Source: three-view drawing plus pictorial views. Frame: mm from the lowest corner of the part. Give positions to 0.01 mm unless a question says otherwise; leave off trailing zeros. Order: outer loops, then holes, each group sorted by start corner. A loop starts at its lowest first (then second) coordinate and runs counter-clockwise, first axis right, second up.
1) First-contact query: P1, Ø13, axis at x = 14.86, z = 35, coming from the +Y side; P2, Ø6, axis at y = 12.5, z = 46, coming from the -X side; P3, Ø10, axis at x = 17.5, y = 14.5, coming from the +Z side; P4, Ø1.5, axis at x = 50, z = 30, coming from the +Y side. Flat tips, straight axial feed; report the tip coordinate or a pass-through.
2) Section C-C, the plane x = 11.5. Return loops of the section in (y, z) (1 decimal).
3) Section B-B, the plane z = 58. Return loops of the section in (x, y) (1 decimal), plus the area to 3 significant figures.
4) Draft query along X for the marked faces 1, 2 and 3. Return one class per face: released by +X, released by -X, zero draft, split by the parting line, or undercut.
5) Section D-D, the plane y = 9.5. Return loops of the section in (x, z) (1 decimal).
6) Section A-A, the plane x = 33.5. Return loops of the section in (y, z) (1 decimal), plus the area to 3 significant figures.
7) Material intervals for line 1 (X direction, y = 11.25, z = 28) (1 decimal); line 2 (Y direction, x = 5, z = 45.5) (1 decimal); line 3 (X direction, y = 8.5, z = 47.5) (1 decimal), sorted ascending.
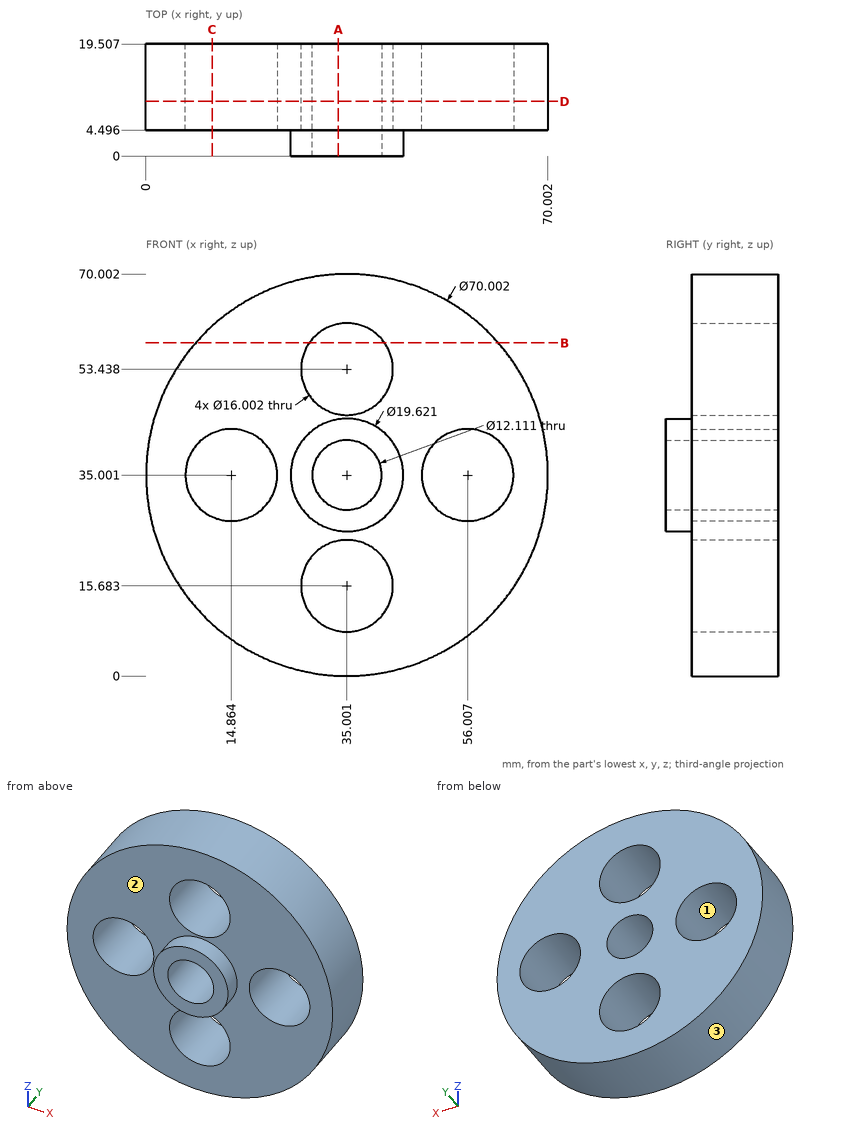
From the geometry:
1. P1: passes through
1. P2: stops at x = 0.93
1. P3: stops at z = 67.69
1. P4: stops at y = 19.51
2. outline: (4.5, 9.1) - (19.5, 9.1) - (19.5, 27.7) - (4.5, 27.7) - close; (4.5, 42.3) - (19.5, 42.3) - (19.5, 60.9) - (4.5, 60.9) - close
3. outline: (8.6, 4.5) - (28.4, 4.5) - (28.4, 19.5) - (8.6, 19.5) - close; (41.6, 4.5) - (61.4, 4.5) - (61.4, 19.5) - (41.6, 19.5) - close
3. area: 595 mm2
4. face 1: undercut
4. face 2: zero draft
4. face 3: split by the parting line
5. outline: circle Ø70 at (35, 35); hole circle Ø16 at (14.9, 35); hole circle Ø16 at (35, 15.7); hole circle Ø16 at (35, 53.4); hole circle Ø12.1 at (35, 35); hole circle Ø16 at (56, 35)
6. outline: (0, 25.3) - (4.5, 25.3) - (4.5, 23.5) - (19.5, 23.5) - (19.5, 29.1) - (0, 29.1) - close; (0, 40.9) - (19.5, 40.9) - (19.5, 45.6) - (4.5, 45.6) - (4.5, 44.7) - (0, 44.7) - close; (4.5, 0) - (19.5, 0) - (19.5, 7.8) - (4.5, 7.8) - close; (4.5, 61.3) - (19.5, 61.3) - (19.5, 70) - (4.5, 70) - close
6. area: 436 mm2
7. line 1: x = 0.7 to 11, 18.7 to 52.1, 59.9 to 69.3
7. line 2: y = 4.5 to 19.5
7. line 3: x = 2.3 to 29.6, 40.4 to 67.7
